Check sheet for the modelled part. Datum: model origin and axes. Units: mm. A direction names the side the tool comes from. Give positions to 0.01 mm unless a question says otherwise; leave off trailing zeros. Order: outer loops, then holes, each group sorted by start corner. A loop starts at its lowest first (then second) coordinate and runs counter-clockwise, first axis right, second up.
from build123d import *

# Parameters (mm, degrees)
SKETCH1_R                     = 1.5
BOSS_EXTRUDE1_DEPTH           = 3
SKETCH4_W                     = 3.5
SKETCH4_H                     = 12
BOSS_EXTRUDE3_DEPTH           = 10.5
SKETCH5_W                     = 2
SKETCH5_H                     = 12
BOSS_EXTRUDE4_DEPTH           = 1.1
SKETCH6_W                     = 0.2
SKETCH6_H                     = 3
BOSS_EXTRUDE5_DEPTH           = 0.5
CHAMFER1_SIZE                 = 10.5
F_3_0MM_DOWEL_HOLE1_D         = 3
F_3_0MM_DOWEL_HOLE1_DEPTH     = 13.5
SKETCH10_R                    = 1.5
BOSS_EXTRUDE6_DEPTH           = 2
CSK_FOR_M3_SFHCS1_D           = 3
CSK_FOR_M3_SFHCS1_DEPTH       = 31.098709071
CSK_FOR_M3_SFHCS1_CSINK_D     = 6.72
CSK_FOR_M3_SFHCS1_CSINK_ANGLE = 90
CSK_FOR_M3_SFHCS1_TIP         = 0.901290929


with BuildPart() as part:
    # Sketch1 → Boss-Extrude1 (new body)
    with BuildSketch(Plane(origin=(0, 0, 0), x_dir=(1, 0, 0), z_dir=(0, 1, 0))):
        with BuildLine():
            Line((-49, 6), (49, 6))
            ThreePointArc((49, 6), (55, 0), (49, -6))
            Line((49, -6), (-49, -6))
            ThreePointArc((-49, -6), (-55, 0), (-49, 6))
        make_face()
        with Locations(Location((-51.5, 0, 0), (0, 0, 270))):
            Circle(SKETCH1_R, mode=Mode.SUBTRACT)
        with Locations(Location((51.5, 0, 0), (0, 0, 270))):
            Circle(SKETCH1_R, mode=Mode.SUBTRACT)
    extrude(amount=BOSS_EXTRUDE1_DEPTH)

    # Sketch4 → Boss-Extrude3 (add)
    with BuildSketch(Plane.XZ):
        with Locations((-21.690023983, 0)):
            Rectangle(SKETCH4_W, SKETCH4_H)
        with Locations((21.690023983, 0)):
            Rectangle(SKETCH4_W, SKETCH4_H)
    extrude(amount=BOSS_EXTRUDE3_DEPTH)

    # Sketch5 → Boss-Extrude4 (add)
    with BuildSketch(Plane.XZ):
        with Locations((5, 0)):
            Rectangle(SKETCH5_W, SKETCH5_H)
        Rectangle(SKETCH5_W, SKETCH5_H)
        with Locations((10, 0)):
            Rectangle(SKETCH5_W, SKETCH5_H)
        with Locations((-5, 0)):
            Rectangle(SKETCH5_W, SKETCH5_H)
        with Locations((-10, 0)):
            Rectangle(SKETCH5_W, SKETCH5_H)
    extrude(amount=BOSS_EXTRUDE4_DEPTH)

    # Sketch6 → Boss-Extrude5 (add)
    with BuildSketch(Plane.XY.offset(6)):
        with Locations((48.9, 1.5)):
            Rectangle(SKETCH6_W, SKETCH6_H)
        with Locations((-48.9, 1.5)):
            Rectangle(SKETCH6_W, SKETCH6_H)
    extrude(amount=BOSS_EXTRUDE5_DEPTH)

    # Chamfer1
    chamfer1_edges = [part.edges().sort_by_distance(p)[0] for p in [
        (23.440023983, 0, 0),
        (-23.440023983, 0, 0),
    ]]
    chamfer(chamfer1_edges, length=CHAMFER1_SIZE - 0.0001)  # a hair under: the kernel refuses the full size

    # Ø3.0mm Dowel Hole1
    with Locations(Plane(origin=(0, 3, 0), x_dir=(1, 0, 0), z_dir=(0, 1, 0))):
        with Locations((-51.5, 0), (51.5, 0)):
            Hole(F_3_0MM_DOWEL_HOLE1_D / 2, depth=F_3_0MM_DOWEL_HOLE1_DEPTH)

    # Sketch10 → Boss-Extrude6 (add)
    with BuildSketch(Plane(origin=(0, 3, 0), x_dir=(1, 0, 0), z_dir=(0, 1, 0))):
        with BuildLine():
            Line((-49, -6), (-49, -6.5))
            Line((-49, -6.5), (-48.8, -6.5))
            Line((-48.8, -6.5), (-48.8, -6))
            Line((-48.8, -6), (48.8, -6))
            Line((48.8, -6), (48.8, -6.5))
            Line((48.8, -6.5), (49, -6.5))
            Line((49, -6.5), (49, -6))
            ThreePointArc((49, -6), (55, 0), (49, 6))
            Line((49, 6), (-49, 6))
            ThreePointArc((-49, 6), (-55, 0), (-49, -6))
        make_face()
        with Locations(Location((-51.5, 0, 0), (0, 0, 270))):
            Circle(SKETCH10_R, mode=Mode.SUBTRACT)
        with Locations(Location((51.5, 0, 0), (0, 0, 270))):
            Circle(SKETCH10_R, mode=Mode.SUBTRACT)
    extrude(amount=BOSS_EXTRUDE6_DEPTH)

    # CSK for M3 SFHCS1
    with Locations(Plane(origin=(0, 5, 0), x_dir=(1, 0, 0), z_dir=(0, 1, 0))):
        with Locations((51.5, 0), (-51.5, 0)):
            CounterSinkHole(CSK_FOR_M3_SFHCS1_D / 2, CSK_FOR_M3_SFHCS1_CSINK_D / 2, depth=CSK_FOR_M3_SFHCS1_DEPTH, counter_sink_angle=CSK_FOR_M3_SFHCS1_CSINK_ANGLE)
            with Locations((0, 0, -(CSK_FOR_M3_SFHCS1_DEPTH + CSK_FOR_M3_SFHCS1_TIP / 2))):  # 118° drill point
                Cone(0, CSK_FOR_M3_SFHCS1_D / 2, CSK_FOR_M3_SFHCS1_TIP, mode=Mode.SUBTRACT)


solid = part.part
1) Draft check along X on faces 1 (the face through (28.62, -5.32, -0.08)), 2 (the face through (-44, 0, 0)), 3 (the face through (-10, -1.1, 0)). Enter one of: +X half, -X half, draft (parallel to the pull), parting line (faces both ways), or undercut.
Recorded:
face 1: +X half
face 2: draft
face 3: undercut
2) Depth check by flat-ended pin: pin 1 Ø3 at (y, z) = (-5.5, -3.5) entering from +X; pin 2 Ø2.5 at (x, z) = (2, 2.5) entering from -Y; pin 3 Ø0.9 at (x, z) = (-2.5, 1) entering from -Y. Enter the tip coordinate at first touch or a pass-through.
Recorded:
pin 1: stops at x = 29.94
pin 2: stops at y = -1.1
pin 3: stops at y = 0
3) Section check C-C, the plane y = -8. Record the cut outline in (x, z), then the cut area to 3 significant figures.
Recorded:
outline: (-25.94, -6) - (-19.94, -6) - (-19.94, 6) - (-25.94, 6) - close; (19.94, -6) - (25.94, -6) - (25.94, 6) - (19.94, 6) - close
area: 144 mm2
4) Material ranges on L1, parallel to X at y = 2.55, z = 0; L2, parallel to Z at x = -8, y = 2.25; L3, parallel to Z at x = 51.5, y = 1.8, recorded low to high.
Recorded:
L1: x = -55 to -53, -50 to 50, 53 to 55
L2: z = -6 to 6
L3: z = -5.45 to -1.5, 1.5 to 5.45
5) Set-up check for faces 4 (the face through (44, 0, 0)), 5 (the face through (19.94, -5, 0)), 6 (the face through (-1, 1, 6)), 7 (the face through (-53, 2, 0)): record each of +Z, -Z, +X, -X, +Y, -Y from which the full face is reachable in a straight line by a thin tool's end or side.
Recorded:
face 4: +Z, -Z, +X, -Y
face 5: +Z, -Z, -Y
face 6: +Z, +Y, -Y
face 7: +Y, -Y
6) Section check B-B, the plane x = -51.5. Record the cut outline in (y, z), then the cut area to 3 significant figures.
Recorded:
outline: (0, -5.45) - (5, -5.45) - (5, -3.36) - (3.14, -1.5) - (0, -1.5) - close; (0, 1.5) - (3.14, 1.5) - (5, 3.36) - (5, 5.45) - (0, 5.45) - close
area: 36.1 mm2
7) Section check A-A, the plane y = 1.5. Record the cut outline in (x, z), then the cut area to 3 significant figures.
Recorded:
outline: (-49, -6) - (49, -6) arc R6 ccw to (49, 6) - (49, 6.5) - (48.8, 6.5) - (48.8, 6) - (-48.8, 6) - (-48.8, 6.5) - (-49, 6.5) - (-49, 6) arc R6 ccw to start; hole circle Ø3 at (-51.5, 0); hole circle Ø3 at (51.5, 0)
area: 1,280 mm2
